Build history of the part. All positions in model axes, mm. Face numbers are marked on the shaded views. A direction names the side the tool comes from. Give positions to 0.01 mm unless a question says otherwise; leave off trailing zeros. Order: outer loops, then holes, each group sorted by start corner. A loop starts at its lowest first (then second) coordinate and runs counter-clockwise, first axis right, second up. Notation, with made-up numbers: (-27, 40) - (-4, 40) arc R16 ccw to (-4, 69) - close; hole circle Ø9 at (14.25, 28.25). An arc over 180 degrees is marked (long way). Use a Markdown table: item, result. Add a question column.
(1) Wall check: line 1 (Z direction, x = 325.5, y = -40); line 2 (X direction, y = -96, z = 6.5). Give the ranges that are in metal, low to high.
(2) Slice it at D-D (x = 270). Write the cut outline in (y, z), then the cut area to 3 significant figures.
(3) Slice it at C-C (z = 10). Write the cut outline in (x, y), then the cut area to 3 significant figures.
(4) Which spindle directions (+Z, -Z, +X, -X, +Y, -Y) get a long thin tool onto all of the face, cutting with end or side? Do the marked faces 1 and 2. Say none if no direction does.
(5) Slice it at A-A (x = 115). Write the cut outline in (y, z).
(6) Slice it at B-B (y = -87). Write the cut outline in (x, z) (3 decimals).
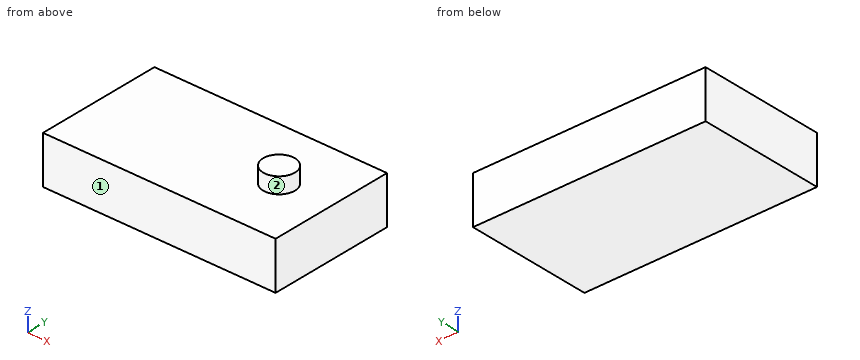
from build123d import *

# Parameters (mm, degrees)
F0_W     = 372.745
F0_H     = 76.2
F1_DEPTH = 203.2
F2_R     = 25.4
F3_DEPTH = 25.4


with BuildPart() as f1:
    # F0 (on Front) → F1 (new body)
    with BuildSketch(Plane.XZ):
        with Locations((186.3725, -38.1)):
            Rectangle(F0_W, F0_H)
    extrude(amount=F1_DEPTH)

    # F2 (on face) → F3 (join)
    with BuildSketch(Plane.XY):
        with Locations((291.115373, -103.962786)):
            Circle(F2_R)
    extrude(amount=F3_DEPTH)


solid = f1.part
Solution:
| question | item | result |
|---|---|---|
| 1 | line 1 | -76.2 to 0 |
| 1 | line 2 | 267 to 315.23 |
| 2 | outline | (-203.2, -76.2) - (0, -76.2) - (0, 0) - (-89.85, 0) - (-89.85, 25.4) - (-118.08, 25.4) - (-118.08, 0) - (-203.2, 0) - close |
| 2 | area | 16,200 mm2 |
| 3 | outline | circle Ø50.8 at (291.12, -103.96) |
| 3 | area | 2,030 mm2 |
| 4 | face 1 | +Z, -Z, +X, -X, -Y |
| 4 | face 2 | +Z |
| 5 | outline | (-203.2, -76.2) - (0, -76.2) - (0, 0) - (-203.2, 0) - close |
| 6 | outline | (0, -76.2) - (372.745, -76.2) - (372.745, 0) - (310.021, 0) - (310.021, 25.4) - (272.21, 25.4) - (272.21, 0) - (0, 0) - close |
